```python
from build123d import *

# Parameters (mm, degrees)
F0_R     = 47.852278
F1_DEPTH = 7.62
F2_T     = -2.54
F4_R     = 5.608286
F4_R_2   = 5.177589
F4_R_3   = 5.217798
F4_R_4   = 5.97792
F4_R_5   = 4.935933
F4_R_6   = 4.445249
F4_R_7   = 4.745595
F4_R_8   = 4.142937
F4_R_9   = 2.93605
F4_R_10  = 4.544521
F4_R_11  = 7.671855
F4_R_12  = 3.835925
F5_DEPTH = 1.27
F6_R     = 5.08


with BuildPart() as f1:
    # F0 (on Front) → F1 (new body)
    with BuildSketch(Plane.XZ):
        with Locations((-75.713672, 36.766488)):
            Circle(F0_R)
    extrude(amount=F1_DEPTH)

    # F2
    f2_openings = [f1.faces().sort_by_distance(p)[0] for p in [
        (-75.713672, -7.62, 36.766488),
    ]]
    offset(amount=F2_T, openings=f2_openings)

    # F4 (on face) → F5 (join)
    with BuildSketch(Plane.XZ.offset(2.54)):
        with Locations((-110.339284, 50.251123)):
            Circle(F4_R)
        with Locations((-112.003483, 24.109663)):
            Circle(F4_R_2)
        with Locations((-85.477225, 5.647067)):
            Circle(F4_R_3)
        with Locations((-59.536304, 12.006708)):
            Circle(F4_R_4)
        with Locations((-59.57577, 37.714168)):
            Circle(F4_R_5)
        with Locations((-40.702716, 29.041462)):
            Circle(F4_R_6)
        with Locations((-90.947576, 27.981274)):
            Circle(F4_R_7)
        with Locations((-90.947576, 70.743375)):
            Circle(F4_R_8)
        with Locations((-77.989683, 75.85264)):
            Circle(F4_R_9)
        with Locations((-75.023986, 65.913238)):
            Circle(F4_R_10)
        with Locations((-53.647552, 62.852636)):
            Circle(F4_R_11)
        with Locations((-65.233916, 53.533848)):
            Circle(F4_R_12)
    extrude(amount=F5_DEPTH)

    # F6
    f6_edges = [f1.edges().sort_by_distance(p)[0] for p in [
        (-123.565949, 0, 36.766488),
    ]]
    fillet(f6_edges, radius=F6_R)


solid = f1.part
```
For this review, take the finished solid that the model builds, in its own axes (mm). A direction names the side the tool comes from. Round coordinates to 2 decimals unless told otherwise and drop trailing zeros. Write each loop counter-clockwise with the first axis right and the second up, starting at its lowest first coordinate (ties: lowest second). Pieces come first, ordered by that corner, then holes. Notation, with made-up numbers: (79.25, 44) -> (96.25, 44) arc R27 cw to (96.25, 68) -> close; hole circle Ø7 at (85.5, -7.75). An arc over 180 degrees is marked (long way). Use one line per item in the form item = value.
1) To check wall thickness, follow L1, parallel to X at y = -2.75, z = 64; L2, parallel to X at y = -2.75, z = 6.5; L3, parallel to Z at x = -89.5, y = -3.75. State the ranges of each line that lie inside material, in increasing order. Write a range as from..to.
Found:
L1 = -114.37..-111.93, -79.15..-70.9, -61.23..-46.06, -39.5..-37.06
L2 = -112.04..-109.44, -90.62..-80.33, -61.86..-57.21, -41.99..-39.38
L3 = -8.87..-6.4, 2.32..8.97, 23.46..32.5, 66.86..74.63, 79.93..82.4
2) Take a section at A-A, the plane y = -6.25. Write out the cut boundary in (x, z), and give its area (3 significant figures).
Found:
outline = circle Ø95.7 at (-75.71, 36.77); hole circle Ø90.62 at (-75.71, 36.77)
area = 743 mm2
3) Tool access review of faces 4 (the cylindrical face through (-49.52, -3.17, 69.32)), 5 (the flat face through (-76, 0, 37)): name each direction out of +Z, -Z, +X, -X, +Y, -Y from which nothing blocks a thin tool from reaching the whole face with its end or side.
Found:
face_4 = -Y
face_5 = +Z, -Z, +X, -X, +Y
4) Clearance check with flat-ended pins moving along their axes: pin 1 (5.5 mm diameter, centred on x = -110, z = 50.5, fed in from -Y); pin 2 (3 mm diameter, centred on x = -105.5, y = -1.5, fed in from +Z); pin 3 (3 mm diameter, centred on x = -106.5, y = -6.5, fed in from +Z). State where each tip first meets the part, or that it passes through.
Found:
pin_1 = -3.81
pin_2 = 74.2
pin_3 = 74.61
5) Mouldability with a two-part tool opening along Z and no side actions: class faces 1 (the flat face through (-76, -2.54, 37)), 2 (the cylindrical face through (-110.98, -6.33, 69.11)), 3 (the flat face through (-40, -7.62, 65)) as +Z half, -Z half, draft (parallel to the pull), parting line (faces both ways), or undercut.
Found:
face_1 = undercut
face_2 = parting line
face_3 = draft
